```python
from build123d import *

# Parameters (mm, degrees)
SKETCH1_W           = 30
SKETCH1_H           = 30
BOSS_EXTRUDE1_DEPTH = 30
SKETCH2_W           = 10
SKETCH2_H           = 10
BOSS_EXTRUDE2_DEPTH = 152.4
SKETCH3_W           = 6
SKETCH3_H           = 6
CUT_EXTRUDE1_DEPTH  = 152.4
SKETCH6_R           = 4.5
CUT_EXTRUDE2_DEPTH  = 15
SKETCH7_R           = 6.7
CUT_EXTRUDE3_DEPTH  = 20
FILLET1_R           = 1.5


with BuildPart() as part:
    # Sketch1 → Boss-Extrude1 (new body)
    with BuildSketch(Plane(origin=(0, 0, 0), x_dir=(0, 0, -1), z_dir=(1, 0, 0))):
        with Locations((-2.320508076, 15)):
            Rectangle(SKETCH1_W, SKETCH1_H)
    boss_extrude1 = extrude(amount=BOSS_EXTRUDE1_DEPTH)

    # Sketch2 → Boss-Extrude2 (add)
    with BuildSketch(Plane(origin=(30, 0, 0), x_dir=(0, 0, -1), z_dir=(1, 0, 0))):
        with Locations((-2.320508076, 15)):
            Rectangle(SKETCH2_W, SKETCH2_H)
    extrude(amount=BOSS_EXTRUDE2_DEPTH)

    # Sketch3 → Cut-Extrude1 (cut)
    with BuildSketch(Plane(origin=(182.4, 0, 0), x_dir=(0, 0, -1), z_dir=(1, 0, 0))):
        with Locations((-2.320508076, 15)):
            Rectangle(SKETCH3_W, SKETCH3_H)
    extrude(amount=-CUT_EXTRUDE1_DEPTH, mode=Mode.SUBTRACT)

    # Sketch6 → Cut-Extrude2 (cut)
    with BuildSketch(Plane(origin=(0, 0, -12.679491924), x_dir=(-1, 0, 0), z_dir=(0, 0, -1))):
        with Locations(Location((-10, 15, 0), (0, 0, 90))):
            Circle(SKETCH6_R)
    cut_extrude2 = extrude(amount=-CUT_EXTRUDE2_DEPTH, mode=Mode.SUBTRACT)

    # Sketch7 → Cut-Extrude3 (cut)
    with BuildSketch(Plane(origin=(0, 27.990381057, -16.160254038), x_dir=(-1, 0, 0), z_dir=(0, 0.8660254037844349, -0.5000000000000066))):
        with Locations(Location((-20, 14.019237886, 0), (0, 0, 90))):
            Circle(SKETCH7_R)
    cut_extrude3 = extrude(amount=-CUT_EXTRUDE3_DEPTH, mode=Mode.SUBTRACT)

    # Mirror1: Boss-Extrude1, Cut-Extrude2, Cut-Extrude3 across plane
    add(boss_extrude1.mirror(Plane(origin=(106.2, 0, 0), x_dir=(0, 0, 1), z_dir=(1, 0, 0))))
    add(cut_extrude2.mirror(Plane(origin=(106.2, 0, 0), x_dir=(0, 0, 1), z_dir=(1, 0, 0))), mode=Mode.SUBTRACT)
    add(cut_extrude3.mirror(Plane(origin=(106.2, 0, 0), x_dir=(0, 0, 1), z_dir=(1, 0, 0))), mode=Mode.SUBTRACT)

    # Fillet1
    fillet1_edges = [part.edges().sort_by_distance(p)[0] for p in [
        (30, 0, 2.320508076),
        (30, 15, 7.320508076),
        (106.2, 20, 7.320508076),
        (30, 10, 2.320508076),
        (106.2, 10, 7.320508076),
        (30, 15, -2.679491924),
        (106.2, 10, -2.679491924),
        (30, 20, 2.320508076),
        (106.2, 20, -2.679491924),
        (30, 15, -12.679491924),
        (182.4, 15, 7.320508076),
        (182.4, 10, 2.320508076),
        (182.4, 15, -2.679491924),
        (182.4, 20, 2.320508076),
        (106.2, 12, -0.679491924),
        (30, 30, 2.320508076),
        (0, 15, -12.679491924),
        (0, 0, 2.320508076),
        (0, 15, 17.320508076),
        (182.4, 30, 2.320508076),
        (197.4, 30, 17.320508076),
        (212.4, 15, -12.679491924),
        (197.4, 30, -12.679491924),
        (182.4, 0, 2.320508076),
        (197.4, 0, -12.679491924),
        (182.4, 15, 17.320508076),
        (197.4, 0, 17.320508076),
        (182.4, 15, -12.679491924),
        (212.4, 30, 2.320508076),
        (212.4, 15, 17.320508076),
        (212.4, 0, 2.320508076),
        (0, 30, 2.320508076),
        (15, 30, -12.679491924),
        (15, 0, -12.679491924),
        (15, 0, 17.320508076),
        (15, 30, 17.320508076),
        (30, 15, 17.320508076),
    ]]
    fillet(fillet1_edges, radius=FILLET1_R)


solid = part.part
```
Geometry check sheet. Reference: the model listing, model coordinates, mm. A direction names the side the tool comes from. Round coordinates to 2 decimals unless told otherwise and drop trailing zeros. Loops run counter-clockwise (first coordinate to the right, second up) from the corner with the lowest first, then second, coordinate; pieces in that order, holes last. Notation, with made-up numbers: M 57.5,52.5 L 72.5,52.5 A18 ccw 72.5,85.5 Z; hole C -9,9 d3. An arc over 180 degrees is marked long. Return JSON: item names as keys, results as strings. Group by question number.
(1) Mould release check, pull along X, two halves, no side actions. Record for faces 1 (the face through (212.4, 15, 3)), 2 (the face through (206.79, 14.02, -5.28)), 3 (the face through (15, 0, 3)): pulls with the +X half, pulls with the -X half, needs draft (parallel to the pull), parting line crosses it, or undercut.
(2) Set-up check for faces 4 (the face through (12, 30, 3)), 5 (the face through (30, 9.2, -3.5)), 6 (the face through (105, 15, -2.679)), 7 (the face through (202, 15, 2.321)), 8 (the face through (105, 20, 2)): record each of +Z, -Z, +X, -X, +Y, -Y from which the full face is reachable in a straight line by a thin tool's end or side.
(3) Go/stop test with flat-tipped pins: pin 1 (7.5 mm diameter, centred on x = 92.5, z = 4, fed in from +Y); pin 2 (2 mm diameter, centred on x = 98.5, z = 3, fed in from -Y); pin 3 (2 mm diameter, centred on x = 78.5, y = 13.5, fed in from -Z); pin 4 (7 mm diameter, centred on x = 204, y = 14, fed in from -Z). Record where each tip stops, or that it passes through.
(4) Scan lines: line 1 along X through (y, z) = (15, -7); line 2 along X through (y, z) = (15, -0.75); line 3 along X through (y, z) = (18.75, 6). Record each from-to range of solid material in increasing order. Write a range as [from, to].
(5) Section check A-A, the plane y = 3.5. Enter the section's corners in (x, z).
(6) Section check B-B, the plane x = 202.4. Enter the section's corners in (y, z).
(7) Section check C-C, the plane x = 136.5. Enter the section's corners in (y, z), and give its area (3 significant figures).
Data:
{
 "1": {"face 1": "pulls with the +X half", "face 2": "undercut", "face 3": "needs draft"},
 "2": {"face 4": "+Z, -Z, +X, -X, +Y", "face 5": "none", "face 6": "-Z, +Y, -Y", "face 7": "-Z", "face 8": "+Z, -Z, +Y"},
 "3": {"pin 1": "y = 20", "pin 2": "y = 10", "pin 3": "z = -2.68", "pin 4": "z = -12.68"},
 "4": {"line 1": "[0, 5.5], [14.5, 30], [182.4, 197.9], [206.9, 212.4]", "line 2": "[0, 5.5], [14.5, 197.9], [206.9, 212.4]", "line 3": "[0, 13.32], [26.68, 185.72], [199.08, 212.4]"},
 "5": {"outline": "M 0,-11.18 A1.5 ccw 1.5,-12.68 L 28.5,-12.68 A1.5 ccw 30,-11.18 L 30,15.82 A1.5 ccw 28.5,17.32 L 1.5,17.32 A1.5 ccw 0,15.82 Z; M 182.4,-11.18 A1.5 ccw 183.9,-12.68 L 210.9,-12.68 A1.5 ccw 212.4,-11.18 L 212.4,15.82 A1.5 ccw 210.9,17.32 L 183.9,17.32 A1.5 ccw 182.4,15.82 Z"},
 "6": {"outline": "M 0,-11.18 A1.5 ccw 1.5,-12.68 L 10.5,-12.68 L 10.5,2.32 L 19.5,2.32 L 19.5,-12.68 L 28.5,-12.68 A1.5 ccw 30,-11.18 L 30,15.82 A1.5 ccw 28.5,17.32 L 1.5,17.32 A1.5 ccw 0,15.82 Z"},
 "7": {"outline": "M 10,-1.18 A1.5 ccw 11.5,-2.68 L 18.5,-2.68 A1.5 ccw 20,-1.18 L 20,5.82 A1.5 ccw 18.5,7.32 L 11.5,7.32 A1.5 ccw 10,5.82 Z; hole M 12,0.82 A1.5 ccw 13.5,-0.68 L 18,-0.68 L 18,5.32 L 12,5.32 Z", "area": "62.6 mm²"}
}
